```python
from build123d import *

# Parameters (mm, degrees)
CYLINDER345_R               = 3.5
CYLINDER345_DEPTH           = 20
CYLINDER339_R               = 1.5
CYLINDER339_DEPTH           = 10
CYLINDER339_PLACEMENT_ANGLE = 67.5
CYLINDER340_R               = 1.5
CYLINDER340_DEPTH           = 10
CYLINDER340_PLACEMENT_ANGLE = 112.5
CYLINDER343_R               = 1.5
CYLINDER343_DEPTH           = 10
CYLINDER343_PLACEMENT_ANGLE = 157.5
CYLINDER341_R               = 1.5
CYLINDER341_DEPTH           = 10
CYLINDER341_PLACEMENT_ANGLE = 202.5
CYLINDER338_R               = 1.5
CYLINDER338_DEPTH           = 10
CYLINDER338_PLACEMENT_ANGLE = 112.500001
CYLINDER344_R               = 1.5
CYLINDER344_DEPTH           = 10
CYLINDER344_PLACEMENT_ANGLE = 67.5
CYLINDER342_R               = 1.5
CYLINDER342_DEPTH           = 10
CYLINDER342_PLACEMENT_ANGLE = 22.5
CYLINDER337_R               = 1.5
CYLINDER337_DEPTH           = 10
CYLINDER337_PLACEMENT_ANGLE = 22.5
TUBE033_R                   = 52
TUBE033_R_2                 = 42
TUBE033_DEPTH               = 1


with BuildPart() as obj1:
    # Cylinder345 → Cylinder345 (new body)
    with BuildSketch(Plane(origin=(-52.3, 0, 29), x_dir=(1, 0, 0), z_dir=(0, 0, 1))):
        Circle(CYLINDER345_R)
    extrude(amount=CYLINDER345_DEPTH)


with BuildPart() as obj2:
    # Cylinder339 → Cylinder339 (new body)
    with BuildSketch(Plane.XY):
        Circle(CYLINDER339_R)
    extrude(amount=CYLINDER339_DEPTH)


with BuildPart() as obj2_1:
    # Cylinder339 placement: moved
    add(obj2.part.moved(Location((44.346218, -18.368805, 35.5))).rotate(Axis((44.346218, -18.368805, 35.5), (0, 0, 1)), CYLINDER339_PLACEMENT_ANGLE))


with BuildPart() as obj3:
    # Cylinder340 → Cylinder340 (new body)
    with BuildSketch(Plane.XY):
        Circle(CYLINDER340_R)
    extrude(amount=CYLINDER340_DEPTH)


with BuildPart() as obj3_1:
    # Cylinder340 placement: moved
    add(obj3.part.moved(Location((44.346218, 18.368805, 35.5))).rotate(Axis((44.346218, 18.368805, 35.5), (0, 0, 1)), CYLINDER340_PLACEMENT_ANGLE))


with BuildPart() as obj4:
    # Cylinder343 → Cylinder343 (new body)
    with BuildSketch(Plane.XY):
        Circle(CYLINDER343_R)
    extrude(amount=CYLINDER343_DEPTH)


with BuildPart() as obj4_1:
    # Cylinder343 placement: moved
    add(obj4.part.moved(Location((18.368805, 44.346218, 35.5))).rotate(Axis((18.368805, 44.346218, 35.5), (0, 0, 1)), CYLINDER343_PLACEMENT_ANGLE))


with BuildPart() as obj5:
    # Cylinder341 → Cylinder341 (new body)
    with BuildSketch(Plane.XY):
        Circle(CYLINDER341_R)
    extrude(amount=CYLINDER341_DEPTH)


with BuildPart() as obj5_1:
    # Cylinder341 placement: moved
    add(obj5.part.moved(Location((-18.368805, 44.346218, 35.5))).rotate(Axis((-18.368805, 44.346218, 35.5), (0, 0, 1)), CYLINDER341_PLACEMENT_ANGLE))


with BuildPart() as obj6:
    # Cylinder338 → Cylinder338 (new body)
    with BuildSketch(Plane.XY):
        Circle(CYLINDER338_R)
    extrude(amount=CYLINDER338_DEPTH)


with BuildPart() as obj6_1:
    # Cylinder338 placement: moved
    add(obj6.part.moved(Location((-44.346218, 18.368805, 35.5))).rotate(Axis((-44.346218, 18.368805, 35.5), (0, 0, -1)), CYLINDER338_PLACEMENT_ANGLE))


with BuildPart() as obj7:
    # Cylinder344 → Cylinder344 (new body)
    with BuildSketch(Plane.XY):
        Circle(CYLINDER344_R)
    extrude(amount=CYLINDER344_DEPTH)


with BuildPart() as obj7_1:
    # Cylinder344 placement: moved
    add(obj7.part.moved(Location((-44.346218, -18.368805, 35.5))).rotate(Axis((-44.346218, -18.368805, 35.5), (0, 0, -1)), CYLINDER344_PLACEMENT_ANGLE))


with BuildPart() as obj8:
    # Cylinder342 → Cylinder342 (new body)
    with BuildSketch(Plane.XY):
        Circle(CYLINDER342_R)
    extrude(amount=CYLINDER342_DEPTH)


with BuildPart() as obj8_1:
    # Cylinder342 placement: moved
    add(obj8.part.moved(Location((-18.368805, -44.346218, 35.5))).rotate(Axis((-18.368805, -44.346218, 35.5), (0, 0, -1)), CYLINDER342_PLACEMENT_ANGLE))


with BuildPart() as compound253:
    # Cylinder337 → Cylinder337 (new body)
    with BuildSketch(Plane.XY):
        Circle(CYLINDER337_R)
    extrude(amount=CYLINDER337_DEPTH)


with BuildPart() as compound253_1:
    # Cylinder337 placement: moved
    add(compound253.part.moved(Location((18.368805, -44.346218, 35.5))).rotate(Axis((18.368805, -44.346218, 35.5), (0, 0, 1)), CYLINDER337_PLACEMENT_ANGLE))

    # Compound253: union obj2, obj3, obj4, obj5, obj6, obj7, obj8
    add(obj2_1.part)
    add(obj3_1.part)
    add(obj4_1.part)
    add(obj5_1.part)
    add(obj6_1.part)
    add(obj7_1.part)
    add(obj8_1.part)


with BuildPart() as compound253_2:
    # Compound253 placement: moved
    add(compound253_1.part.moved(Location((0, 0, -2))))


with BuildPart() as cut143:
    # Tube033 → Tube033 (new body)
    with BuildSketch(Plane.XY.offset(37)):
        Circle(TUBE033_R)
        Circle(TUBE033_R_2, mode=Mode.SUBTRACT)
    extrude(amount=TUBE033_DEPTH)

    # Cut142: cut Compound253
    add(compound253_2.part, mode=Mode.SUBTRACT)

    # Cut143: cut obj1
    add(obj1.part, mode=Mode.SUBTRACT)


solid = cut143.part
```
For this review, take the finished solid that the model builds, in its own axes (mm). Coordinates: 2 decimals unless noted, no trailing zeros. Order: outer loops, then holes, each group sorted by start corner. A loop starts at its lowest first (then second) coordinate and runs counter-clockwise, first axis right, second up. Notation, with made-up numbers: (31.25, 84.25) - (51.25, 84.25) arc R16 cw to (51.25, 88.25) - close; hole circle Ø7 at (-3.5, 22). An arc over 180 degrees is marked (long way). Answer as a JSON object with one key per item and string values. Group by question number.
1. We need section B-B on x = 0. State the section outline as (y, z) points.
2. We need section A-A on y = 0. State the section outline as (x, z) points.
3. For probe 1 along X at (y, z) = (-18, 37.85); probe 2 along X at (y, z) = (-14, 37.65); probe 3 along X at (y, z) = (-1, 37.85), list the stretches that pass through material, from the lowest coordinate up.
4. We need section C-C on z = 37.65. Give the number of separate pieces and of enclosed holes in the cut face, then the cut area to 3 significant figures.
5. The part is to be moulded in two halves that separate along X. For faces 1 (the flat face through (-4, -42, 37)), 2 (the cylindrical face through (17.98, 42.897, 37.493)), 3 (the cylindrical face through (-48.8, -0.1, 37.5)), say which applies: pulls with the +X half, pulls with the -X half, needs draft (parallel to the pull), parting line crosses it, or undercut.
Final values:
{
 "1": {"outline": "(-52, 37) - (-42, 37) - (-42, 38) - (-52, 38) - close; (42, 37) - (52, 37) - (52, 38) - (42, 38) - close"},
 "2": {"outline": "(-48.8, 37) - (-42, 37) - (-42, 38) - (-48.8, 38) - close; (42, 37) - (52, 37) - (52, 38) - (42, 38) - close"},
 "3": {"probe 1": "-48.79 to -45.8, -42.89 to -37.95, 37.95 to 42.89, 45.8 to 48.79", "probe 2": "-50.08 to -39.6, 39.6 to 50.08", "probe 3": "-48.95 to -41.99, 41.99 to 51.99"},
 "4": {"separate pieces": "1", "enclosed holes": "9", "area": "2,880 mm²"},
 "5": {"face 1": "needs draft", "face 2": "undercut", "face 3": "pulls with the -X half"}
}
